Read the model definition and answer for the solid it produces. Units are mm, in the model's axes. Face numbers are marked on the shaded views. Coordinates: 2 decimals unless noted, no trailing zeros. Order: outer loops, then holes, each group sorted by start corner. A loop starts at its lowest first (then second) coordinate and runs counter-clockwise, first axis right, second up. Notation, with made-up numbers: M 40.25,34.5 L 48.25,34.5 A7 cw 48.25,46.5 Z; hole C -3,7 d4. An arc over 180 degrees is marked long. One line per question, with ' | ' between items. Start each with the question number.
1) Find section B-B, the plane y = 14.5. Write down the section's boundary in (x, z).
2) The mould has two halves that part along X. Classify the marked faces 1, 2 and 3: +X half, -X half, draft (parallel to the pull), parting line (faces both ways), or undercut.
3) Find section C-C, the plane x = 109. Write down the section's boundary in (y, z), plus the area to 3 significant figures.
4) Find section A-A, the plane x = 159. Write down the section's boundary in (y, z).
5) Find section D-D, the plane z = 7. Write down the section's boundary in (x, y).
6) Consider probe 1 along X at (y, z) = (3.25, 10.25); probe 2 along X at (y, z) = (3.25, 1.7); probe 3 along Y at (x, z) = (44.5, -7). Determine where each line is inside the solid, lowest interval first.
7) Given P1, Ø2.5, axis at x = -5.5, y = 10.5, coming from the +Z side; P2, Ø7.5, axis at y = 12, z = 8.5, coming from the +X side; P3, Ø10, axis at x = 150, y = 6, coming from the -Z side; P4, Ø7, axis at x = -4.5, z = 9.5, coming from the +Y side, each flat-ended and moving along its own axis, determine where each tip first touches the part or whether it passes through.
from build123d import *

# Parameters (mm, degrees)
BOSS_EXTRUDE1_DEPTH                          = 175
FILLET1_R                                    = 8
CSK_FOR_M3_COUNTERSUNK_FLAT_HEAD_SCR_2_COUNT = 2
CSK_FOR_M3_COUNTERSUNK_FLAT_HEAD_SCR_2_PITCH = 129
CSK_FOR_M3_COUNTERSUNK_FLAT_HEAD_SCR_3_COUNT = 2
CSK_FOR_M3_COUNTERSUNK_FLAT_HEAD_SCR_3_PITCH = 86
CSK_FOR_M3_COUNTERSUNK_FLAT_HEAD_SCR_4_COUNT = 2
CSK_FOR_M3_COUNTERSUNK_FLAT_HEAD_SCR_4_PITCH = 43
CUT_EXTRUDE2_DEPTH                           = 177.259042321
SKETCH8_W                                    = 12.5
SKETCH8_H                                    = 10
CUT_EXTRUDE3_DEPTH                           = 177.896156092
SKETCH10_W                                   = 8
SKETCH10_H                                   = 18
BOSS_EXTRUDE2_DEPTH                          = 1.5
BOSS_EXTRUDE3_DEPTH                          = 18.5
FILLET2_R                                    = 0.65


with BuildPart() as part:
    # Sketch1 → Boss-Extrude1 (new body)
    with BuildSketch(Plane(origin=(0, 0, 0), x_dir=(0, 0, -1), z_dir=(1, 0, 0))):
        Polygon((0, 6.5), (-25, 0), (-25, -1.5), (10, -1.5), (10, 0), (0, 0), align=None)
    extrude(amount=BOSS_EXTRUDE1_DEPTH)

    # Fillet1
    # the kernel refuses this fillet: 8 mm, written as the material it takes off along each edge
    with BuildSketch(Plane(origin=(-10.545555265, 0, 25), x_dir=(0, 0.2516338517649508, -0.967822506788272), z_dir=(1, 0, 0))) as fillet1_piece_1:
        with BuildLine():
            CenterArc((4.218222106, -8), FILLET1_R, 90, 35.061762164)
            Line((-0.377450778, -1.45173376), (-0.469364235, -1.320768435))
            ThreePointArc((-0.469364235, -1.320768435), (-0.34357699, -0.685605464), (-0.154851601, 0.040261416))
            Line((-0.154851601, 0.040261416), (0, 0.16))
            Line((0, 0.16), (4.218222106, 0.16))
            Line((4.218222106, 0.16), (4.218222106, 0))
        make_face()
    extrude(amount=196.091110529, mode=Mode.SUBTRACT)

    # Sketch5 → CSK for M3 Countersunk Flat Head Screw1 (revolve, cut)
    with BuildSketch(Plane(origin=(152, 3.25, 5), x_dir=(0, -1, 0), z_dir=(1, 0, 0))):
        Polygon((0, 0), (0, 15), (1.7, 15), (1.7, 1.45), (3.15, 0), align=None)
    csk_for_m3_countersunk_flat_head_screw1 = revolve(axis=Axis((152, 3.25, 11.35), (0, 0, -1)), mode=Mode.SUBTRACT)

    # CSK for M3 Countersunk Flat Head Scr 2: CSK for M3 Countersunk Flat Head Screw1 ×2
    with Locations(*[(-i * CSK_FOR_M3_COUNTERSUNK_FLAT_HEAD_SCR_2_PITCH, 0, 0) for i in range(1, CSK_FOR_M3_COUNTERSUNK_FLAT_HEAD_SCR_2_COUNT)]):
        add(csk_for_m3_countersunk_flat_head_screw1, mode=Mode.SUBTRACT)

    # CSK for M3 Countersunk Flat Head Scr 3: CSK for M3 Countersunk Flat Head Screw1 ×2
    with Locations(*[(-i * CSK_FOR_M3_COUNTERSUNK_FLAT_HEAD_SCR_3_PITCH, 0, 0) for i in range(1, CSK_FOR_M3_COUNTERSUNK_FLAT_HEAD_SCR_3_COUNT)]):
        add(csk_for_m3_countersunk_flat_head_screw1, mode=Mode.SUBTRACT)

    # CSK for M3 Countersunk Flat Head Scr 4: CSK for M3 Countersunk Flat Head Screw1 ×2
    with Locations(*[(-i * CSK_FOR_M3_COUNTERSUNK_FLAT_HEAD_SCR_4_PITCH, 0, 0) for i in range(1, CSK_FOR_M3_COUNTERSUNK_FLAT_HEAD_SCR_4_COUNT)]):
        add(csk_for_m3_countersunk_flat_head_screw1, mode=Mode.SUBTRACT)

    # Sketch7 → Cut-Extrude2 (cut, through all)
    with BuildSketch(Plane(origin=(0, 0, 5), x_dir=(-1, 0, 0), z_dir=(0, 0, -1))):
        with BuildLine():
            Line((-149.526136625, 5.2), (-154.473863375, 5.2))
            ThreePointArc((-154.473863375, 5.2), (-152, 0.1), (-149.526136625, 5.2))
        make_face()
        with BuildLine():
            Line((-20.526136625, 5.2), (-25.473863375, 5.2))
            ThreePointArc((-25.473863375, 5.2), (-23, 0.1), (-20.526136625, 5.2))
        make_face()
        with BuildLine():
            Line((-63.526136625, 5.2), (-68.473863375, 5.2))
            ThreePointArc((-68.473863375, 5.2), (-66, 0.1), (-63.526136625, 5.2))
        make_face()
        with BuildLine():
            Line((-106.526136625, 5.2), (-111.473863375, 5.2))
            ThreePointArc((-111.473863375, 5.2), (-109, 0.1), (-106.526136625, 5.2))
        make_face()
    extrude(amount=-CUT_EXTRUDE2_DEPTH, mode=Mode.SUBTRACT)

    # Sketch8 → Cut-Extrude3 (cut, through all)
    with BuildSketch(Plane(origin=(0, 0, 0), x_dir=(1, 0, 0), z_dir=(0, 1, 0))):
        with Locations((6.25, 5)):
            Rectangle(SKETCH8_W, SKETCH8_H)
    extrude(amount=-CUT_EXTRUDE3_DEPTH, mode=Mode.SUBTRACT)

    # Sketch10 → Boss-Extrude2 (add)
    with BuildSketch(Plane.XZ.offset(1.5)):
        with Locations((-4, 9)):
            Rectangle(SKETCH10_W, SKETCH10_H)
    extrude(amount=-BOSS_EXTRUDE2_DEPTH)

    # Sketch11 → Boss-Extrude3 (add)
    with BuildSketch(Plane(origin=(0, 0, 0), x_dir=(1, 0, 0), z_dir=(0, 1, 0))):
        Polygon((-6.52, -15.05), (-6.52, 0), (-8, 0), (-8, -18), (0, -18), (0, -15.05), align=None)
    extrude(amount=BOSS_EXTRUDE3_DEPTH)

    # Fillet2
    fillet2_edges = [part.edges().sort_by_distance(p)[0] for p in [
        (87.5, -1.5, 25),
    ]]
    fillet(fillet2_edges, radius=FILLET2_R)


solid = part.part
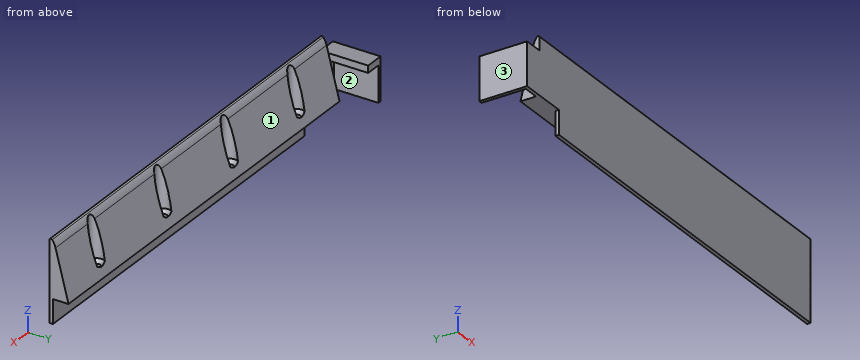
Report:
1) outline: M -8,0 L -6.52,0 L -6.52,15.05 L 0,15.05 L 0,18 L -8,18 Z
2) face 1: draft | face 2: undercut | face 3: -X half
3) outline: M -1.5,-10 L 0,-10 L 0,0 L 1.55,0 L 1.55,3.55 L 0.1,5 L 0.1,23.15 A8 ccw -0.33,23.77 A0.65 ccw -1.5,23.38 Z; M 4.95,0 L 6.5,0 L 5.45,4.05 L 4.95,3.55 Z | area: 63.3 mm^2
4) outline: M -1.5,-10 L 0,-10 L 0,0 L 6.5,0 L 1.06,20.92 A8 ccw -0.33,23.77 A0.65 ccw -1.5,23.38 Z
5) outline: M -8,-1.5 L 175,-1.5 L 175,4.68 L 154.81,4.68 A3.15 cw long 149.19,4.68 L 111.81,4.68 A3.15 cw long 106.19,4.68 L 68.81,4.68 A3.15 cw long 63.19,4.68 L 25.81,4.68 A3.15 cw long 20.19,4.68 L 0,4.68 L 0,0 L -6.52,0 L -6.52,18.5 L -8,18.5 Z
6) probe 1: x = -8 to -6.52, 0 to 19.85, 26.15 to 62.85, 69.15 to 105.85, 112.15 to 148.85, 155.15 to 175 | probe 2: x = -8 to -6.52, 0 to 21.3, 24.7 to 64.3, 67.7 to 107.3, 110.7 to 150.3, 153.7 to 175 | probe 3: y = -1.5 to 0
7) P1: stops at z = 18 | P2: stops at x = -6.52 | P3: stops at z = 0 | P4: stops at y = 18.5
